```python
from build123d import *

# Parameters (mm, degrees)
F1_DEPTH = 15
F2_R     = 3
F3_DEPTH = 15.001
F4_W     = 3
F4_H     = 7
F5_DEPTH = 10
F6_R     = 2
F7_DEPTH = 5


with BuildPart() as f1:
    # F0 (on Front) → F1 (new body)
    with BuildSketch(Plane.XZ):
        with BuildLine():
            Line((15.5, 15), (1, 15))
            ThreePointArc((1, 15), (0.292893, 14.707107), (0, 14))
            Line((0, 14), (0, 1))
            ThreePointArc((0, 1), (0.292893, 0.292893), (1, 0))
            Line((1, 0), (15.5, 0))
            Line((15.5, 0), (15.5, 3))
            ThreePointArc((15.5, 3), (15.93934, 4.06066), (17, 4.5))
            Line((17, 4.5), (30, 4.5))
            Line((30, 4.5), (30, 10.5))
            Line((30, 10.5), (17, 10.5))
            ThreePointArc((17, 10.5), (15.93934, 10.93934), (15.5, 12))
            Line((15.5, 12), (15.5, 15))
        make_face()
        with BuildLine():
            ThreePointArc((10.001502, 4.75), (7.25, 7.501527), (10.004555, 10.249996))
            Line((10.004555, 10.249996), (10.99999, 10.25))
            ThreePointArc((10.99999, 10.25), (12.94454, 9.444547), (13.75, 7.5))
            ThreePointArc((13.75, 7.5), (12.967788, 5.578982), (11.066137, 4.750795))
            ThreePointArc((11.066137, 4.750795), (11.002054, 4.750001), (10.937969, 4.7507))
            Line((10.937969, 4.7507), (10.001502, 4.75))
        make_face(mode=Mode.SUBTRACT)
    extrude(amount=F1_DEPTH)

    # F2 (on Top) → F3 (cut, through all)
    with BuildSketch(Plane.XY):
        with Locations((24, -7.846627)):
            Circle(F2_R)
    extrude(amount=F3_DEPTH, mode=Mode.SUBTRACT)

    # F4 (on face) → F5 (cut)
    with BuildSketch(Plane(origin=(0, 0, 0), x_dir=(-1, 0, 0), z_dir=(0, 1, 0))):
        with Locations((-6.5, 7.5)):
            Rectangle(F4_W, F4_H)
    extrude(amount=-F5_DEPTH, mode=Mode.SUBTRACT)

    # F6 (on face) → F7 (cut)
    with BuildSketch(Plane(origin=(0, 0, 0), x_dir=(0, -1, 0), z_dir=(-1, 0, 0))):
        with Locations((6, 7.5)):
            Circle(F6_R)
    extrude(amount=-F7_DEPTH, mode=Mode.SUBTRACT)


solid = f1.part
```
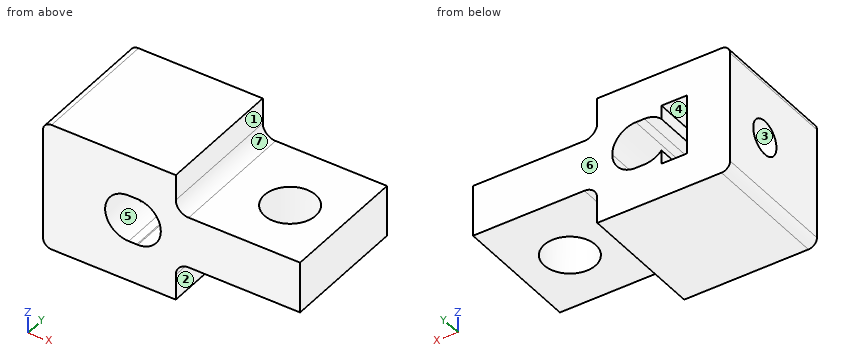
Input: part model. Units: mm. Frame: model coordinates. Face numbers are marked on the shaded views. A direction names the side the tool comes from. Give positions to 0.01 mm unless a question says otherwise; leave off trailing zeros. Loops run counter-clockwise (first coordinate to the right, second up) from the corner with the lowest first, then second, coordinate; pieces in that order, holes last. Notation, with made-up numbers: (-12, 26) -> (11, 26) arc R19 cw to (11, 48) -> close; hole circle Ø6 at (87.5, -33.75). An arc over 180 degrees is marked (long way). Use a Markdown table: item, result.
Q1. Section query D-D, the plane y = -13. Return the cut outline in (x, z), plus the area to 3 significant figures.
Entries:
| item | result |
|---|---|
| outline | (0, 1) arc R1 ccw to (1, 0) -> (15.5, 0) -> (15.5, 3) arc R1.5 cw to (17, 4.5) -> (30, 4.5) -> (30, 10.5) -> (17, 10.5) arc R1.5 cw to (15.5, 12) -> (15.5, 15) -> (1, 15) arc R1 ccw to (0, 14) -> close; hole (10, 4.75) -> (10.94, 4.75) arc R2.75 ccw to (11.07, 4.75) arc R2.75 ccw to (11, 10.25) -> (10, 10.25) arc R2.75 ccw to start |
| area | 291 mm² |
Q2. Pull-direction query (X, two-part tool) for the marked faces 5, 6 and 7; classes: pulls with the +X half, pulls with the -X half, needs draft (parallel to the pull), parting line crosses it, or undercut.
Entries:
| item | result |
|---|---|
| face 5 | undercut |
| face 6 | needs draft |
| face 7 | pulls with the +X half |
Q3. Access query for the marked faces 1, 2, 3 and 4. Directions: +Z, -Z, +X, -X, +Y, -Y. A direction counts if a zero-diameter tool reaches every point of the face in a straight line with its end or side. Return the directions, or none.
Entries:
| item | result |
|---|---|
| face 1 | +Z, +X, +Y, -Y |
| face 2 | -Z, +X, +Y, -Y |
| face 3 | -X |
| face 4 | +Y |
Q4. Ray query, probe 1 along Y at (x, z) = (24, 7.8); probe 2 along Z at (x, y) = (3.9, -6); probe 3 along Z at (x, y) = (11, -12). Return the intervals inside material, ascending. Write a range as from..to.
Entries:
| item | result |
|---|---|
| probe 1 | y = -15..-10.85, -4.85..0 |
| probe 2 | z = 0..5.5, 9.5..15 |
| probe 3 | z = 0..4.75, 10.25..15 |
Q5. Section query B-B, the plane y = -1.5. Return the cut outline in (x, z), plus the area to 3 significant figures.
Entries:
| item | result |
|---|---|
| outline | (0, 1) arc R1 ccw to (1, 0) -> (15.5, 0) -> (15.5, 3) arc R1.5 cw to (17, 4.5) -> (30, 4.5) -> (30, 10.5) -> (17, 10.5) arc R1.5 cw to (15.5, 12) -> (15.5, 15) -> (1, 15) arc R1 ccw to (0, 14) -> close; hole (5, 4) -> (8, 4) -> (8, 5.61) arc R2.75 ccw to (10, 4.75) -> (10.94, 4.75) arc R2.75 ccw to (11.07, 4.75) arc R2.75 ccw to (11, 10.25) -> (10, 10.25) arc R2.75 ccw to (8, 9.39) -> (8, 11) -> (5, 11) -> close |
| area | 272 mm² |
Q6. Section query A-A, the plane x = 24. Return the cut outline in (y, z), plus the area to 3 significant figures.
Entries:
| item | result |
|---|---|
| outline | (-15, 4.5) -> (-10.85, 4.5) -> (-10.85, 10.5) -> (-15, 10.5) -> close; (-4.85, 4.5) -> (0, 4.5) -> (0, 10.5) -> (-4.85, 10.5) -> close |
| area | 54.0 mm² |
Q7. First-contact query: P1, Ø3.5, axis at y = -6.5, z = 2, coming from the +X side; P2, Ø2.5, axis at y = -6, z = 7.5, coming from the -X side; P3, Ø4, axis at x = 23, y = -6, coming from the -Z side. Flat tips, straight axial feed; report the tip coordinate or a pass-through.
Entries:
| item | result |
|---|---|
| P1 | stops at x = 15.7 |
| P2 | stops at x = 13.45 |
| P3 | stops at z = 4.5 |
